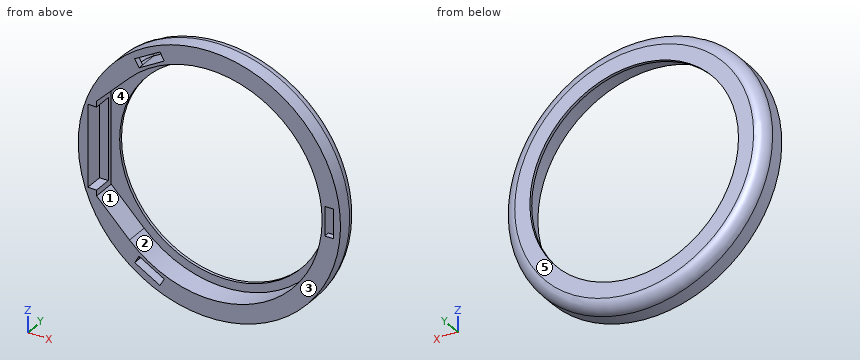
```python
from build123d import *

# Parameters (mm, degrees)
SKETCH1_R           = 22.5
BOSS_EXTRUDE1_DEPTH = 4.5
SKETCH2_R           = 17.9
CUT_EXTRUDE1_DEPTH  = 33.136427928
CUT_EXTRUDE2_DEPTH  = 4
SKETCH4_W           = 1.5
SKETCH4_H           = 14
CUT_EXTRUDE3_DEPTH  = 3.2
FILLET2_R           = 2
SKETCH5_W           = 1.5
SKETCH5_H           = 5
CUT_EXTRUDE4_DEPTH  = 4
SKETCH6_R           = 1.5
CUT_EXTRUDE5_DEPTH  = 1.5
SKETCH7_R           = 1.5
CUT_EXTRUDE6_DEPTH  = 1.5
SKETCH8_R           = 1.5
CUT_EXTRUDE7_DEPTH  = 1.5


with BuildPart() as part:
    # Sketch1 → Boss-Extrude1 (new body)
    with BuildSketch(Plane(origin=(0, 0, 0), x_dir=(1, 0, 0), z_dir=(0, 1, 0))):
        with Locations(Location((0, 0, 0), (0, 0, 270))):
            Circle(SKETCH1_R)
    extrude(amount=BOSS_EXTRUDE1_DEPTH)

    # Sketch2 → Cut-Extrude1 (cut, through all)
    with BuildSketch(Plane(origin=(0, 4.5, 0), x_dir=(1, 0, 0), z_dir=(0, 1, 0))):
        with Locations(Location((0, 0, 0), (0, 0, 270))):
            Circle(SKETCH2_R)
    extrude(amount=-CUT_EXTRUDE1_DEPTH, mode=Mode.SUBTRACT)

    # Sketch3 → Cut-Extrude2 (cut)
    with BuildSketch(Plane.XZ):
        with BuildLine():
            Line((-13.700654905, -13.664353449), (-19.35, -8))
            Line((-19.35, -8), (-19.35, 8))
            Line((-19.35, 8), (-13.700654905, 13.664353449))
            ThreePointArc((-13.700654905, 13.664353449), (19.35, 0), (-13.700654905, -13.664353449))
        make_face()
    extrude(amount=-CUT_EXTRUDE2_DEPTH, mode=Mode.SUBTRACT)

    # Sketch4 → Cut-Extrude3 (cut)
    with BuildSketch(Plane.XZ):
        with Locations((-20.1, 0)):
            Rectangle(SKETCH4_W, SKETCH4_H)
    extrude(amount=-CUT_EXTRUDE3_DEPTH, mode=Mode.SUBTRACT)

    # Fillet2
    fillet2_edges = [part.edges().sort_by_distance(p)[0] for p in [
        (0, 4.5, -22.5),
    ]]
    fillet(fillet2_edges, radius=FILLET2_R)

    # Sketch5 → Cut-Extrude4 (cut)
    with BuildSketch(Plane.XZ):
        Polygon((-12.815063509, 17.196341101), (-12.065063509, 15.897302995), (-7.734936491, 18.397302995), (-8.484936491, 19.696341101), align=None)
        with Locations((20.55, 0)):
            Rectangle(SKETCH5_W, SKETCH5_H)
        Polygon((-12.815063509, -17.196341101), (-8.484936491, -19.696341101), (-7.734936491, -18.397302995), (-12.065063509, -15.897302995), align=None)
    extrude(amount=-CUT_EXTRUDE4_DEPTH, mode=Mode.SUBTRACT)

    # Sketch6 → Cut-Extrude5 (cut)
    with BuildSketch(Plane(origin=(-9.9, 0, 17.147302995), x_dir=(0.8660254037844397, 0, 0.4999999999999981), z_dir=(-0.4999999999999981, 0, 0.8660254037844397))):
        with Locations((2.5, 2.5)):
            Circle(SKETCH6_R)
        with Locations((-2.5, 2.5)):
            Circle(SKETCH6_R)
    extrude(amount=CUT_EXTRUDE5_DEPTH, mode=Mode.SUBTRACT)

    # Sketch7 → Cut-Extrude6 (cut)
    with BuildSketch(Plane(origin=(-9.9, 0, -17.147302995), x_dir=(-0.8660254037844364, 0, 0.500000000000004), z_dir=(-0.500000000000004, 0, -0.8660254037844365))):
        with Locations((-2.5, 2.5)):
            Circle(SKETCH7_R)
        with Locations((2.5, 2.5)):
            Circle(SKETCH7_R)
    extrude(amount=CUT_EXTRUDE6_DEPTH, mode=Mode.SUBTRACT)

    # Sketch8 → Cut-Extrude7 (cut)
    with BuildSketch(Plane(origin=(19.8, 0, 0), x_dir=(0, 0, -1), z_dir=(1, 0, 0))):
        with Locations((2.5, 2.5)):
            Circle(SKETCH8_R)
        with Locations((-2.5, 2.5)):
            Circle(SKETCH8_R)
    extrude(amount=CUT_EXTRUDE7_DEPTH, mode=Mode.SUBTRACT)


solid = part.part
```
Part model, mm, in its own coordinate system. Face numbers are marked on the shaded views. A direction names the side the tool comes from. Give positions to 0.01 mm unless a question says otherwise; leave off trailing zeros. Order: outer loops, then holes, each group sorted by start corner. A loop starts at its lowest first (then second) coordinate and runs counter-clockwise, first axis right, second up. Notation, with made-up numbers: (26, 75.5) - (35, 75.5) arc R13 ccw to (35, 93.5) - close; hole circle Ø3 at (81.25, 54.5). An arc over 180 degrees is marked (long way). Use one line per item in the form item = value.
Item 1: Slice it at B-B on z = 0. Give the cut face in (x, y).
Solution:
outline = (-22.5, 0) - (-20.85, 0) - (-20.85, 3.2) - (-19.35, 3.2) - (-19.35, 4) - (-17.9, 4) - (-17.9, 4.5) - (-20.5, 4.5) arc R2 ccw to (-22.5, 2.5) - close; (17.9, 4) - (19.35, 4) - (19.35, 0) - (19.8, 0) - (19.8, 4) - (21.3, 4) - (21.3, 0) - (22.5, 0) - (22.5, 2.5) arc R2 ccw to (20.5, 4.5) - (17.9, 4.5) - close
Item 2: Two-plate mould, pull along X, no slides. Class the marked faces 1, 2 and 3: released by +X, released by -X, zero draft, split by the parting line, or undercut.
Solution:
face_1 = undercut
face_2 = undercut
face_3 = zero draft
Item 3: Slice it at A-A on x = 0. Give the cut face in (y, z), and give its area (3 significant figures).
Solution:
outline = (0, -22.5) - (2.5, -22.5) arc R2 ccw to (4.5, -20.5) - (4.5, -17.9) - (4, -17.9) - (4, -19.35) - (0, -19.35) - close; (0, 19.35) - (4, 19.35) - (4, 17.9) - (4.5, 17.9) - (4.5, 20.5) arc R2 ccw to (2.5, 22.5) - (0, 22.5) - close
area = 28.1 mm2
Item 4: Which spindle directions (+Z, -Z, +X, -X, +Y, -Y) get a long thin tool onto all of the face, cutting with end or side? Do the marked faces 4 and 5. Say none if no direction does.
Solution:
face_4 = -Y
face_5 = +Z, -Z, +X, -X, +Y
Item 5: Pin check, flat tips, straight feed: pin 1 Ø1.6 at (x, y) = (-20.5, 1) entering from -Z; pin 2 Ø2 at (x, y) = (-5, 3.5) entering from -Z; pin 3 Ø1 at (y, z) = (1.5, 1.5) entering from +X. Stop position of each tip, or through.
Solution:
pin_1 = -10.87
pin_2 = -22.07
pin_3 = 22.48
Item 6: Probe probe 1 along Z at (x, y) = (-11.5, 3.15); probe 2 along Z at (x, y) = (12.5, 1.4); probe 3 along X at (y, z) = (0.3, 11). List the from-to ranges inside material, lowest first. Write a range as from..to.
Solution:
probe_1 = -19.21..-17.96, -16.22..-15.56, 15.56..16.22, 17.96..19.21
probe_2 = -18.71..-14.77, 14.77..18.71
probe_3 = -19.63..-16.36, 15.92..19.63
